Answer from the drawing. Dimensions are ordinates in mm from the lowest x, y and z of the part. A direction names the side the tool comes from. Coordinates: 2 decimals unless noted, no trailing zeros. Write each loop counter-clockwise with the first axis right and the second up, starting at its lowest first coordinate (ties: lowest second). Pieces come first, ordered by that corner, then holes.
(1) For a pull along Y with two mould halves and no side action, classify the marked faces 4, 5 and 6 as +Y half, -Y half, draft (parallel to the pull), parting line (faces both ways), or undercut.
(2) The part is cut by section D-D on x = 58.42. Determine the outline of the cut face in (y, z).
(3) Which of the six approach directions +Z, -Z, +X, -X, +Y, -Y give full straight-line access (tool end or side, diameter ignored) to the marked faces 1, 2 and 3?
(4) Given P1, Ø3, axis at y = 16.5, z = 8, coming from the -X side; P2, Ø6.5, axis at x = 44.45, y = 6.35, coming from the +Z side; P3, Ø4, axis at x = 44.45, y = 36.83, coming from the +Z side; P4, Ø4, axis at x = 9.5, z = 8, coming from the -Y side, each flat-ended and moving along its own axis, determine where each tip first touches the part or whether it passes through.
(5) The part is cut by section C-C on z = 8.75. Give the number of separate pieces and of enclosed holes in the cut face, plus the area to 3 significant figures.
(6) The part is cut by section A-A on x = 6.35. Determine the outline of the cut face in (y, z).
(7) Straight lines are drawn through the part: line 1 (Y direction, x = 58.42, z = 3.25); line 2 (Y direction, x = 6.35, z = 5.5); line 3 (Y direction, x = 42.5, z = 7.5) (1 decimal). For each, find the intervals that lie inside material, in ascending order.
(8) The part is cut by section B-B on y = 44.45. Determine the outline of the cut face in (x, z), plus the area to 3 significant figures.
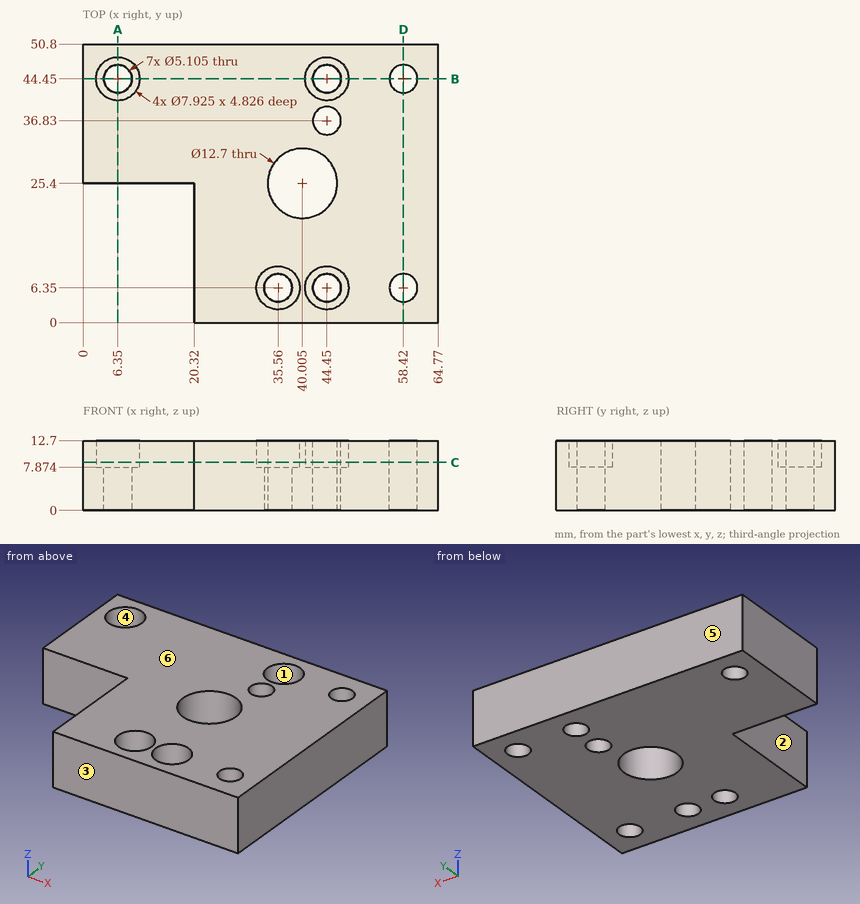
Model answer:
1. face 4: undercut
1. face 5: +Y half
1. face 6: draft
2. outline: (0, 0) - (3.8, 0) - (3.8, 12.7) - (0, 12.7) - close; (8.9, 0) - (41.9, 0) - (41.9, 12.7) - (8.9, 12.7) - close; (47, 0) - (50.8, 0) - (50.8, 12.7) - (47, 12.7) - close
3. face 1: +Z
3. face 2: +Z, -Z, -X, -Y
3. face 3: +Z, -Z, +X, -X, -Y
4. P1: stops at x = 20.32
4. P2: stops at z = 7.87
4. P3: passes through
4. P4: stops at y = 25.4
5. separate pieces: 1
5. enclosed holes: 8
5. area: 2,390 mm2
6. outline: (25.4, 0) - (41.9, 0) - (41.9, 7.87) - (40.49, 7.87) - (40.49, 12.7) - (25.4, 12.7) - close; (47, 0) - (50.8, 0) - (50.8, 12.7) - (48.41, 12.7) - (48.41, 7.87) - (47, 7.87) - close
7. line 1: y = 0 to 3.8, 8.9 to 41.9, 47 to 50.8
7. line 2: y = 25.4 to 41.9, 47 to 50.8
7. line 3: y = 0 to 4.7, 8 to 19.6, 31.2 to 35.2, 38.5 to 42.8, 46.1 to 50.8
8. outline: (0, 0) - (3.8, 0) - (3.8, 7.87) - (2.39, 7.87) - (2.39, 12.7) - (0, 12.7) - close; (8.9, 0) - (41.9, 0) - (41.9, 7.87) - (40.49, 7.87) - (40.49, 12.7) - (10.31, 12.7) - (10.31, 7.87) - (8.9, 7.87) - close; (47, 0) - (55.87, 0) - (55.87, 12.7) - (48.41, 12.7) - (48.41, 7.87) - (47, 7.87) - close; (60.97, 0) - (64.77, 0) - (64.77, 12.7) - (60.97, 12.7) - close
8. area: 601 mm2
